Geometry check sheet. Reference: the model listing, model coordinates, mm. Round coordinates to 2 decimals unless told otherwise and drop trailing zeros. Write each loop counter-clockwise with the first axis right and the second up, starting at its lowest first coordinate (ties: lowest second). Pieces come first, ordered by that corner, then holes. Notation, with made-up numbers: M -5.5,79.25 L 28.5,79.25 A12 ccw 28.5,101.25 Z; hole C 78,-10.5 d6. An arc over 180 degrees is marked long. Answer as CSV lines item,"result". Start each with the question number.
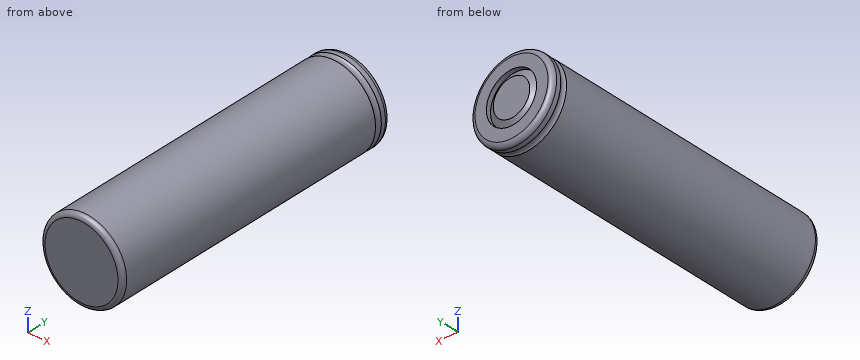
```python
from build123d import *

# Parameters (mm, degrees)
FILLET2_R = 1


with BuildPart() as part:
    # Sketch2 → Revolve1 (revolve)
    with BuildSketch(Plane.XY, mode=Mode.PRIVATE) as revolve1_sk:
        with BuildLine():
            Line((0, 0), (9, 0))
            Line((9, 0), (9, 61.585786438))
            ThreePointArc((9, 61.585786438), (8.707106781, 62.292893219), (9, 63))
            Line((9, 63), (9, 65))
            Line((9, 65), (5.5, 65))
            Line((5.5, 65), (5.5, 64))
            Line((5.5, 64), (4, 65))
            Line((4, 65), (0, 65))
            Line((0, 65), (0, 0))
        make_face()
    revolve(revolve1_sk.sketch.rotate(Axis((0, 0, 0), (0, 1, 0)), 90), axis=Axis((0, 0, 0), (0, 1, 0)))

    # Fillet2
    fillet2_edges = [part.edges().sort_by_distance(p)[0] for p in [
        (0, 0, 9),
        (0, 65, 9),
    ]]
    fillet(fillet2_edges, radius=FILLET2_R)


solid = part.part
```
1) Go/stop test with flat-tipped pins: pin 1 (2 mm diameter, centred on x = 3, y = 45, fed in from -Z); pin 2 (4 mm diameter, centred on y = 48.5, z = -7, fed in from +X); pin 3 (4 mm diameter, centred on y = 12.5, z = 4, fed in from +X). Record where each tip stops, or that it passes through.
2) Scan lines: line 1 (X direction, y = 64.35, z = 0) (3 decimals); line 2 (X direction, y = 64.55, z = 0) (3 decimals); line 3 (Y direction, x = -3.5, z = 7.25). Record each from-to range of solid material in increasing order. Write a range as from..to.
3) Section check A-A, the plane y = 26. Record the cut outline in (x, z), plus the area to 3 significant figures.
Results:
1,pin 1,"stops at z = -8.77"
1,pin 2,"stops at x = 7.48"
1,pin 3,"stops at x = 8.77"
2,line 1,"x = -8.937..-5.5, -4.975..4.975, 5.5..8.937"
2,line 2,"x = -8.835..-5.5, -4.675..4.675, 5.5..8.835"
2,line 3,"y = 0..65"
3,outline,"C 0,0 d18"
3,area,"254 mm^2"
